Autodesk Inventor part; units mm, degrees
ref_plane "YZ Plane" through (0, 0, 0) normal (1, 0, 0) x (0, 1, 0)
ref_plane "XZ Plane" through (0, 0, 0) normal (0, 1, 0) x (-1, 0, 0)
ref_plane "XY Plane" through (0, 0, 0) normal (0, 0, 1) x (1, 0, 0)
sketch "Sketch1" plane through (0, 0, 0) normal (0, 1, 0) x (-1, 0, 0)
  arc A0 (-220, 0) -> (-67, -209.5495) centre (0, 0) ccw
  arc A1 (-217, 0) -> (-67, -206.3977) centre (0, 0) ccw
  line L0 (-220, 0) -> (-217, 0)
  line L1 (0, -220) -> (0, -217)
  line L2 (0, -220) -> (-67, -220)
  line L3 (0, -220) -> (67, -220) construction
  line L4 (-67, -220) -> (-67, -206.3977)
  line L5 (-67, -206.3977) -> (-65.0308, -207.0265)
  line L6 (-67, -206.3977) -> (-68.4601, -210.9695)
  point P0 (-67.9127, -209.2555)
  dimension "d0" = 440
  dimension "d1" = 3
  dimension "d2" = 67
  dimension "d3" = 180
  dimension "d9" = 90
extrude "Extrusion1" add sketch "Sketch1" along normal blind 92.5 contours L0 A1 L6 A0
sketch "Sketch2" plane through (0, 0, 0) normal (0, -1, 0) x (1, 0, 0)
  arc A0 (67, -206.3977) -> (217, 0) centre (0, 0) ccw
  arc A1 (60.8249, -187.3748) -> (197, 0) centre (0, 0) ccw
  line L0 (197, 0) -> (217, 0)
  line L1 (60.8249, -187.3748) -> (67, -206.3977)
  dimension "d6" = 20
extrude "Extrusion2" add sketch "Sketch2" against normal blind 3
sketch "Sketch7" plane through (0, 0, 0) normal (0, -1, 0) x (1, 0, 0)
  arc A0 (60.8249, -187.3748) -> (197, 0) centre (0, 0) ccw
  arc A1 (67.9127, -209.2555) -> (220, 0) centre (0, 0) ccw
  line L0 (197, 0) -> (220, 0)
  line L1 (196.9772, -3) -> (219.9795, -3)
  dimension "d28" = 3
extrude "Extrusion6" add sketch "Sketch7" against normal up to surface (92.5 mm away)
sketch "Sketch8" plane through (0, 3, 0) normal (0, 1, 0) x (1, 0, 0)
  arc A0 (196.9772, 3) -> (60.8249, 187.3748) centre (0, 0) ccw
  line L0 (67, 206.3977) -> (60.8249, 187.3748)
  line L1 (67, 206.3977) -> (67, 185.2566)
  line L2 (67, 206.3977) -> (88.1411, 206.3977) construction
  dimension "d31" = 90
extrude "Extrusion7" cut sketch "Sketch8" against normal blind 10
properties part number "Bottom_Enclosure_1"
Read the model definition and answer for the solid it produces. Units are mm, in the model's axes. A direction names the side the tool comes from. Coordinates: 2 decimals unless noted, no trailing zeros. Order: outer loops, then holes, each group sorted by start corner. A loop starts at its lowest first (then second) coordinate and runs counter-clockwise, first axis right, second up. Notation, with made-up numbers: (84.25, 38) -> (107.25, 38) arc R17 cw to (107.25, 49) -> close; hole circle Ø5 at (-26.5, 20). An arc over 180 degrees is marked (long way). Answer as a JSON object with one key per item and string values.
1) Each of these flat-tipped pins is pushed along its axis until it touches: pin 1 (12 mm diameter, centred on x = 203, y = 22, fed in from +Z); pin 2 (8 mm diameter, centred on x = 147.5, y = 26.5, fed in from -Z); pin 3 (10 mm diameter, centred on x = 205.5, y = 51, fed in from -Z); pin 4 (10 mm diameter, centred on x = 160.5, y = 17, fed in from -Z). Where does it stop, or does it pass through?
Model answer:
{"pin 1": "stops at z = 0", "pin 2": "stops at z = -166.76", "pin 3": "stops at z = -90.55", "pin 4": "stops at z = -155.63"}
2) A cutting plane is placed at A-A, the plane x = 204.5. Determine the outline of the cut face in (y, z).
Model answer:
{"outline": "(0, -81.12) -> (92.5, -81.12) -> (92.5, -72.59) -> (3, -72.59) -> (3, -3) -> (92.5, -3) -> (92.5, 0) -> (0, 0) -> close"}
3) The mould has two halves that part along Z. Classify faces 1 (the face through (176.82, 45.6, -130.9)), 2 (the face through (164, 3, -112)), 3 (the face through (184, 92.5, -120)): released by +Z, released by -Z, zero draft, split by the parting line, or undercut.
Model answer:
{"face 1": "released by -Z", "face 2": "undercut", "face 3": "zero draft"}
4) A tool of negligible diameter and unlimited length cuts with its end or side. For faces 4 (the face through (209, 46, 0)), 5 (the face through (207, 47, -3)), from which of +Z, -Z, +X, -X, +Y, -Y can it reach the whole face along a straight path? Write none if from no direction.
Model answer:
{"face 4": "+Z, +X, -X, +Y, -Y", "face 5": "-X, +Y"}
5) Consider line 1 along Y through (x, z) = (99.5, -190); line 2 along X through (y, z) = (71.5, -178.5); line 3 along Z through (x, y) = (147, 75.5). Determine where each line is inside the solid, lowest interval first. Write a range as from..to.
Model answer:
{"line 1": "y = 0..3", "line 2": "x = 123.4..128.6", "line 3": "z = -163.68..-159.62"}
6) A cutting plane is placed at B-B, the plane z = -145.5. Determine the outline of the cut face in (x, y), plus the area to 3 significant figures.
Model answer:
{"outline": "(132.81, 0) -> (165.01, 0) -> (165.01, 92.5) -> (160.99, 92.5) -> (160.99, 3) -> (132.81, 3) -> close", "area": "457 mm²"}
7) A cutting plane is placed at C-C, the plane y = 75.5. Determine the outline of the cut face in (x, z).
Model answer:
{"outline": "(67, -206.4) -> (67.91, -209.26) arc R220 ccw to (220, 0) -> (197, 0) arc R197 cw to (196.98, -3) -> (216.98, -3) arc R217 cw to start"}
